```python
from build123d import *

# Parameters (mm, degrees)
F2_R     = 6.35
F3_DEPTH = 25.4
F4_R     = 25.4
F5_DEPTH = 12.7


with BuildPart() as f1:
    # F0 (on Top) → F1 (revolve)
    with BuildSketch(Plane.XY):
        with BuildLine():
            ThreePointArc((-12.7, 0), (0, -12.7), (12.7, 0))
            Line((12.7, 0), (-12.7, 0))
        make_face()
    revolve(axis=Axis((0, 0, 0), (1, 0, 0)))

    # F2 (on Top) → F3 (join)
    with BuildSketch(Plane.XY):
        Circle(F2_R)
    extrude(amount=F3_DEPTH)

    # F4 (on face) → F5 (join)
    with BuildSketch(Plane.XY.offset(25.4)):
        Circle(F4_R)
    extrude(amount=F5_DEPTH)


solid = f1.part
```
Verification items for the finished model (mm, model axes). Round coordinates to 2 decimals unless told otherwise and drop trailing zeros. Order: outer loops, then holes, each group sorted by start corner. A loop starts at its lowest first (then second) coordinate and runs counter-clockwise, first axis right, second up. Notation, with made-up numbers: (88.25, -14) -> (107.25, -14) arc R32 cw to (107.25, 19) -> close; hole circle Ø2 at (19.5, -2.5). An arc over 180 degrees is marked (long way). Put each result on its own line as item: value. Start each with the question number.
(1) Section check D-D (y = -9). Enter the section's corners in (x, z).
(2) Depth check by flat-ended pin: pin 1 Ø5 at (x, z) = (-20, 25.5) entering from +Y; pin 2 Ø3 at (x, z) = (-2.5, 7.5) entering from +Y; pin 3 Ø8 at (y, z) = (9.5, 26) entering from +X. Enter the tip coordinate at first touch or a pass-through.
(3) Section check C-C (z = 33.5). Enter the section's corners in (x, y), then the cut area to 3 significant figures.
(4) Section check A-A (y = 0). Enter the section's corners in (x, z), then the cut area to 3 significant figures.
(5) Draft check along Z on faces 1 (the face through (0, 0, 38.1)), 2 (the face through (-1.38, -6.2, 18.1)), 3 (the face through (-5.506, -24.796, 31.661)), 4 (the face through (5, -5, 25.4)). Enter one of: +Z half, -Z half, draft (parallel to the pull), parting line (faces both ways), or undercut.
(6) Material ranges on line 1 along Z through (x, y) = (-21, 6); line 2 along Z through (x, y) = (0, -10.5); line 3 along Y through (x, z) = (-0.5, 35.5), recorded low to high.
Completed:
1. outline: (-23.75, 25.4) -> (23.75, 25.4) -> (23.75, 38.1) -> (-23.75, 38.1) -> close; circle Ø17.92 at (0, 0)
2. pin 1: stops at y = 18.41
2. pin 2: stops at y = 10.97
2. pin 3: stops at x = 24.8
3. outline: circle Ø50.8 at (0, 0)
3. area: 2,030 mm2
4. outline: (-25.4, 25.4) -> (-6.35, 25.4) -> (-6.35, 11) arc R12.7 ccw (long way) to (6.35, 11) -> (6.35, 25.4) -> (25.4, 25.4) -> (25.4, 38.1) -> (-25.4, 38.1) -> close
4. area: 1,320 mm2
5. face 1: +Z half
5. face 2: undercut
5. face 3: draft
5. face 4: undercut
6. line 1: z = 25.4 to 38.1
6. line 2: z = -7.14 to 7.14, 25.4 to 38.1
6. line 3: y = -25.4 to 25.4
